from build123d import *

# Parameters (mm, degrees)
SKETCH_1_W         = 28.5
SKETCH_1_H         = 7
BASE_DEPTH         = 1.5
SKETCH_4_R         = 0.725
AXIS_DEPTH         = 1.9
HOLE_WIZARD_M2_1_D = 1.6


with BuildPart() as part:
    # 草图1 → base (new body)
    with BuildSketch(Plane.XY):
        with Locations((3.85, 4.3)):
            Rectangle(SKETCH_1_W, SKETCH_1_H)
    extrude(amount=BASE_DEPTH)

    # 草图4 → axis (add)
    with BuildSketch(Plane(origin=(0, 0, 0), x_dir=(-1, 0, 0), z_dir=(0, 0, -1))):
        with Locations(Location((-11.1, 3.3, 0), (0, 0, 270))):
            Circle(SKETCH_4_R)
    extrude(amount=AXIS_DEPTH)

    # M2 螺纹孔的螺纹孔钻头1 (through all)
    with Locations(Plane(origin=(0.6, 4.05, 0), x_dir=(-1, 0, 0), z_dir=(0, 0, -1))):
        with Locations((0, 0)):
            Hole(HOLE_WIZARD_M2_1_D / 2)


solid = part.part
Could you check a few things on this model? Use its own coordinates, in mm. Coordinates: 2 decimals unless noted, no trailing zeros. Loops run counter-clockwise (first coordinate to the right, second up) from the corner with the lowest first, then second, coordinate; pieces in that order, holes last. Notation, with made-up numbers: (43, 79) -> (90, 79) arc R20 cw to (90, 117) -> close; hole circle Ø2 at (-15, -8.75). An arc over 180 degrees is marked (long way). Answer in a Markdown table with one row per item.
(1) Thinking about a two-plate mould opening in Y: for faces 1 (the face through (4, 4, 0)), 2 (the face through (0.496, 4.843, 0.761)), 3 (the face through (10.49, 2.91, -0.94)), which applies, released by +Y, released by -Y, zero draft, split by the parting line, or undercut?
Results found:
| item | result |
|---|---|
| face 1 | zero draft |
| face 2 | undercut |
| face 3 | split by the parting line |
(2) Imagine slicing it at C-C (z = -0.3). List the corners of the cut face in (x, y) for me (3 decimals), plus the area to 3 significant figures.
Results found:
| item | result |
|---|---|
| outline | circle Ø1.45 at (11.1, 3.3) |
| area | 1.65 mm^2 |
(3) Imagine slicing it at A-A (x = 0.6). List the corners of the cut face in (y, z) for me, plus the area to 3 significant figures.
Results found:
| item | result |
|---|---|
| outline | (0.8, 0) -> (3.25, 0) -> (3.25, 1.5) -> (0.8, 1.5) -> close; (4.85, 0) -> (7.8, 0) -> (7.8, 1.5) -> (4.85, 1.5) -> close |
| area | 8.10 mm^2 |
(4) Imagine slicing it at B-B (x = 11.1). List the corners of the cut face in (y, z) for me (3 decimals), plus the area to 3 significant figures.
Results found:
| item | result |
|---|---|
| outline | (0.8, 0) -> (2.575, 0) -> (2.575, -1.9) -> (4.025, -1.9) -> (4.025, 0) -> (7.8, 0) -> (7.8, 1.5) -> (0.8, 1.5) -> close |
| area | 13.3 mm^2 |
(5) Will this pin go through, and if not, where does the flat tip stop? pin 1 Ø2 at (x, y) = (0.6, 4.05) entering from -Z.
Results found:
| item | result |
|---|---|
| pin 1 | stops at z = 0 |
(6) If I drill on probe 1 along Y at (x, z) = (0.6, 0.3); probe 2 along Z at (x, y) = (-9, 3.75); probe 3 along X at (y, z) = (4.75, 0.9), over which ranges is the centre line in solid material (lowest first)?
Results found:
| item | result |
|---|---|
| probe 1 | y = 0.8 to 3.25, 4.85 to 7.8 |
| probe 2 | z = 0 to 1.5 |
| probe 3 | x = -10.4 to 0.21, 0.99 to 18.1 |
(7) Imagine slicing it at D-D (y = 2). List the corners of the cut face in (x, z) for me.
Results found:
| item | result |
|---|---|
| outline | (-10.4, 0) -> (18.1, 0) -> (18.1, 1.5) -> (-10.4, 1.5) -> close |
